Autodesk Inventor part; units mm, degrees
ref_plane "YZ Plane" through (0, 0, 0) normal (1, 0, 0) x (0, 1, 0)
ref_plane "XZ Plane" through (0, 0, 0) normal (0, 1, 0) x (-1, 0, 0)
ref_plane "XY Plane" through (0, 0, 0) normal (0, 0, 1) x (1, 0, 0)
sketch "Sketch1" plane through (0, 0, 0) normal (0, 0, 1) x (1, 0, 0)
  line L0 (0, 0) -> (25, 0)
  line L1 (25, 0) -> (25, 3)
  line L2 (25, 3) -> (3, 3)
  line L3 (3, 3) -> (3, 25)
  line L4 (3, 25) -> (0, 25)
  line L5 (0, 25) -> (0, 0)
  dimension "d0" = 25
  dimension "d1" = 3
  dimension "d2" = 22
  dimension "d3" = 22
extrude "Extrusion1" add sketch "Sketch1" along normal blind 60
sketch "Sketch2" plane through (3, 3, 0) normal (1, 0, 0) x (0, 0, -1)
  line L0 (0, 0) -> (0, 22)
  line L1 (0, 22) -> (-60, 22)
  line L2 (-60, 0) -> (-60, 22)
  line L3 (0, 0) -> (-60, 0)
  line L4 (0, 22) -> (-1.4085, 22)
  line L5 (0, 22) -> (-9.5, 22) construction
  line L6 (-9.5, 22) -> (-8.5825, 22) construction
  line L7 (-9.5, 22) -> (-23.165, 22) construction
  line L8 (-23.165, 22) -> (-23.165, 2.4653) construction
  point P0 (0, -3)
  dimension "d6" = 9.5
  dimension "d7" = 13.665
properties part number "printed Y rod holder bracket"
The listing builds one solid part. Answer for the finished solid, in the listing's coordinates (mm). A direction names the side the tool comes from. Round coordinates to 2 decimals unless told otherwise and drop trailing zeros. Order: outer loops, then holes, each group sorted by start corner. A loop starts at its lowest first (then second) coordinate and runs counter-clockwise, first axis right, second up. Notation, with made-up numbers: M 13.5,83.25 L 60.5,83.25 A12 ccw 60.5,101.25 Z; hole C 39.25,34.5 d11. An arc over 180 degrees is marked long. Answer in a Markdown table with one row per item. Add a question column.
1) Flat-ended cylindrical pins translate along their axes: pin 1 Ø3 at (y, z) = (16, 10.5) entering from +X; pin 2 Ø6.5 at (x, z) = (12, 27) entering from +Y. Find the tip coordinate at first contact, or state that the pin passes through.
2) The part is cut by section B-B on x = 5.5. Determine the outline of the cut face in (y, z), plus the area to 3 significant figures.
3) Consider line 1 along Y through (x, z) = (11.5, 6). Determine where the line is inside the solid, lowest interval first. Write a range as from..to.
4) The part is cut by section A-A on z = 46. Determine the outline of the cut face in (x, y).
5) Which of the six approach directions +Z, -Z, +X, -X, +Y, -Y give full straight-line access (tool end or side, diameter ignored) to faces 1 (the face through (7, 2, 60)), 2 (the face through (3, 14, 30))?
Findings below:
| question | item | result |
|---|---|---|
| 1 | pin 1 | stops at x = 3 |
| 1 | pin 2 | stops at y = 3 |
| 2 | outline | M 0,0 L 3,0 L 3,60 L 0,60 Z |
| 2 | area | 180 mm² |
| 3 | line 1 | y = 0..3 |
| 4 | outline | M 0,0 L 25,0 L 25,3 L 3,3 L 3,25 L 0,25 Z |
| 5 | face 1 | +Z, +X, -X, +Y, -Y |
| 5 | face 2 | +Z, -Z, +X, +Y |
